Could you check a few things on this model? Use its own coordinates, in mm. A direction names the side the tool comes from. Give positions to 0.01 mm unless a question says otherwise; leave off trailing zeros. Write each loop counter-clockwise with the first axis right and the second up, starting at its lowest first coordinate (ties: lowest second). Pieces come first, ordered by that corner, then holes. Notation, with made-up numbers: (70, 37) - (128, 37) arc R29 cw to (128, 59) - close; hole circle Ø7 at (57.25, -36). An arc over 180 degrees is marked (long way). Write item = value, one per line.
from build123d import *

# Parameters (mm, degrees)
SKETCH1_R          = 5
SKETCH1_R_2        = 2.5
BASE_FLANGE1_DEPTH = 3


# Sheet-metal steps are written as plain solids
with BuildPart() as part:
    # Sketch1 → Base-Flange1 (new body)
    with BuildSketch(Plane.XY):
        with BuildLine():
            Line((-14.238080804, 7.633940989), (-49.730098253, -22.147397762))
            ThreePointArc((-49.730098253, -22.147397762), (-52.365300026, -25.581659576), (-53.302222156, -29.807842194))
            Line((-53.302222156, -29.807842194), (-53.302222156, -48.56164166))
            Line((-53.302222156, -48.56164166), (-53.302222156, -76.139380484))
            ThreePointArc((-53.302222156, -76.139380484), (-51.544862843, -80.382021171), (-47.302222156, -82.139380484))
            Line((-47.302222156, -82.139380484), (-29.302222156, -82.139380484))
            ThreePointArc((-29.302222156, -82.139380484), (-25.059581469, -80.382021171), (-23.302222156, -76.139380484))
            Line((-23.302222156, -76.139380484), (-23.302222156, -48.56164166))
            Line((-23.302222156, -48.56164166), (-23.302222156, -43.797071938))
            ThreePointArc((-23.302222156, -43.797071938), (-22.365300026, -39.570889321), (-19.730098253, -36.136627507))
            Line((-19.730098253, -36.136627507), (5.045547487, -15.347392305))
            ThreePointArc((5.045547487, -15.347392305), (7.165990017, -11.274060103), (5.785088487, -6.894399988))
            Line((5.785088487, -6.894399988), (-5.785088487, 6.894399988))
            ThreePointArc((-5.785088487, 6.894399988), (-9.858420689, 9.014842519), (-14.238080804, 7.633940989))
        make_face()
        with Locations((-38.302222156, -67.139380484)):
            Circle(SKETCH1_R, mode=Mode.SUBTRACT)
        with Locations((-11.490666647, -9.641814145)):
            Circle(SKETCH1_R_2, mode=Mode.SUBTRACT)
        with Locations((-22.981333294, -19.283628291)):
            Circle(SKETCH1_R_2, mode=Mode.SUBTRACT)
    extrude(amount=-BASE_FLANGE1_DEPTH)


solid = part.part
1. If we section it at D-D, the plane y = -45.5: Please give me the cut outline in (x, z), and give its area (3 significant figures).
Filled sheet:
outline = (-53.3, -3) - (-23.3, -3) - (-23.3, 0) - (-53.3, 0) - close
area = 90.0 mm2
2. Thinking about a two-plate mould opening in Y: for faces 3 (the face through (-31.74, -7.05, -1.48)), 4 (the face through (-22.391, -39.626, -1.479)), 5 (the face through (-30, -36, -3)), 6 (the face through (-21.6, -17.2, -1.5)), which applies, pulls with the +Y half, pulls with the -Y half, needs draft (parallel to the pull), parting line crosses it, or undercut?
Filled sheet:
face_3 = pulls with the +Y half
face_4 = pulls with the -Y half
face_5 = needs draft
face_6 = undercut
3. If we section it at C-C, the plane z = -1.8: Please give me the cut outline in (x, y), and give its area (3 significant figures).
Filled sheet:
outline = (-53.3, -76.14) arc R6 ccw to (-47.3, -82.14) - (-29.3, -82.14) arc R6 ccw to (-23.3, -76.14) - (-23.3, -43.8) arc R10 cw to (-19.73, -36.14) - (5.05, -15.35) arc R6 ccw to (5.79, -6.89) - (-5.79, 6.89) arc R6 ccw to (-14.24, 7.63) - (-49.73, -22.15) arc R10 ccw to (-53.3, -29.81) - close; hole circle Ø10 at (-38.3, -67.14); hole circle Ø5 at (-22.98, -19.28); hole circle Ø5 at (-11.49, -9.64)
area = 2,850 mm2
4. If we section it at A-A, the plane y = -20.5: Please give me the cut outline in (x, z).
Filled sheet:
outline = (-47.77, -3) - (-25.17, -3) - (-25.17, 0) - (-47.77, 0) - close; (-20.8, -3) - (-1.1, -3) - (-1.1, 0) - (-20.8, 0) - close
5. I need wall thicknesses on line 1 (Y direction, x = -37, z = -0.7); line 2 (Y direction, x = -12, z = -1.8); line 3 (X direction, y = -49.5, z = -2.05). Which ranges of each line are inside material? Lowest first, please.
Filled sheet:
line_1 = -82.14 to -71.97, -62.31 to -11.47
line_2 = -29.65 to -12.09, -7.19 to 8.82
line_3 = -53.3 to -23.3
6. Which directions (+Z, -Z, +X, -X, +Y, -Y) give clear straight access to the entire face, cutting with the end or side of a thin tool? Please do faces 1 (the face through (-23.302, -60, -1)), 2 (the face through (-13.475, -11.163, -1.479)).
Filled sheet:
face_1 = +Z, -Z, +X, -Y
face_2 = +Z, -Z
7. For pin 1 (1.5 mm diameter, centred on x = -13.5, z = -1.5, fed in from -Y); pin 2 (3 mm diameter, centred on x = -22.98, y = -19.28, fed in from -Z); pin 3 (1.5 mm diameter, centred on y = -5, z = -1.5, fed in from +X); pin 4 (1.5 mm diameter, centred on y = -3.5, z = -1, fed in from +X), each with a flat end and sliding along its axis, tell me the tip position at first contact or that it passes through.
Filled sheet:
pin_1 = -31.54
pin_2 = through
pin_3 = 4.82
pin_4 = 3.57
8. If we section it at B-B, the plane x = -42: Please give me the cut outline in (y, z).
Filled sheet:
outline = (-82.14, -3) - (-70.5, -3) - (-70.5, 0) - (-82.14, 0) - close; (-63.77, -3) - (-15.66, -3) - (-15.66, 0) - (-63.77, 0) - close
